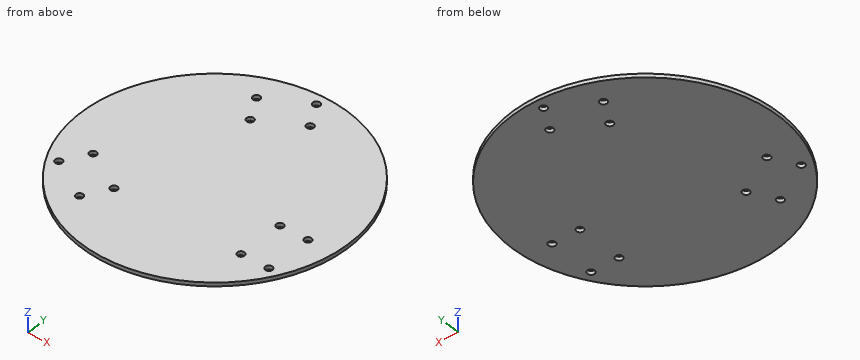
from build123d import *

# Parameters (mm, degrees)
SKETCH_1_R               = 70.710678119
EXTRUDE_1_DEPTH          = 2
SKETCH_2_R               = 1.9
CUT_EXTRUDE_2_DEPTH      = 101.019998
PATTERN_CIRCULAR_1_COUNT = 3


with BuildPart() as part:
    # ｽｹｯﾁ1 → ﾎﾞｽ - 押し出し1 (new body)
    with BuildSketch(Plane.XY):
        Circle(SKETCH_1_R)
    extrude(amount=EXTRUDE_1_DEPTH)

    # ｽｹｯﾁ2 → ｶｯﾄ - 押し出し2 (cut, symmetric)
    with BuildSketch(Plane.XY):
        with Locations((41.18, -7.5)):
            Circle(SKETCH_2_R)
        with Locations((41.18, -32.5)):
            Circle(SKETCH_2_R)
        with Locations((56.18, -32.5)):
            Circle(SKETCH_2_R)
        with Locations((56.18, -7.5)):
            Circle(SKETCH_2_R)
    cut_extrude_2 = extrude(amount=CUT_EXTRUDE_2_DEPTH, both=True, mode=Mode.SUBTRACT)

    # 円形ﾊﾟﾀｰﾝ1: ｶｯﾄ - 押し出し2 ×3 about axis
    pattern_circular_1_axis = Axis((-0.140995034, 0.057927294, 0), (0, 0, 1))
    for i in range(1, PATTERN_CIRCULAR_1_COUNT):
        add(cut_extrude_2.rotate(pattern_circular_1_axis, i * 360 / PATTERN_CIRCULAR_1_COUNT), mode=Mode.SUBTRACT)


solid = part.part
The listing builds one solid part. Answer for the finished solid, in the listing's coordinates (mm). Coordinates: 2 decimals unless noted, no trailing zeros. Loops run counter-clockwise (first coordinate to the right, second up) from the corner with the lowest first, then second, coordinate; pieces in that order, holes last.
1) Find the intervals of material crossed by L1, parallel to X at y = -1, z = 0.65; L2, parallel to Y at x = 41.18, z = 1.45; L3, parallel to Y at x = 56.18, z = 1, in increasing order.
2) A flat-ended cylindrical pin translates along its axis: pin 1 Ø4.5 at (x, y) = (-34.85, -44.94) entering from -Z. Find the tip coordinate at first contact, or state that the pin passes through.
3) Find section C-C on z = 0.9. Give the number of separate pieces and of enclosed holes in the cut face, then the cut area to 3 significant figures.
4) Find section A-A on y = -7.5. Write down the section's boundary in (x, z), then the cut area to 3 significant figures.
5) Find section D-D on x = 15. Write down the section's boundary in (y, z), then the cut area to 3 significant figures.
6) Find section B-B on x = 56.18. Write down the section's boundary in (y, z).
Values:
1. L1: x = -70.7 to 70.7
1. L2: y = -57.48 to -34.4, -30.6 to -9.4, -5.6 to 57.48
1. L3: y = -42.94 to -34.4, -30.6 to -9.4, -5.6 to 42.94
2. pin 1: stops at z = 0
3. separate pieces: 1
3. enclosed holes: 12
3. area: 15,600 mm2
4. outline: (-70.31, 0) - (39.28, 0) - (39.28, 2) - (-70.31, 2) - close; (43.08, 0) - (54.28, 0) - (54.28, 2) - (43.08, 2) - close; (58.08, 0) - (70.31, 0) - (70.31, 2) - (58.08, 2) - close
4. area: 266 mm2
5. outline: (-69.1, 0) - (69.1, 0) - (69.1, 2) - (-69.1, 2) - close
5. area: 276 mm2
6. outline: (-42.94, 0) - (-34.4, 0) - (-34.4, 2) - (-42.94, 2) - close; (-30.6, 0) - (-9.4, 0) - (-9.4, 2) - (-30.6, 2) - close; (-5.6, 0) - (42.94, 0) - (42.94, 2) - (-5.6, 2) - close
